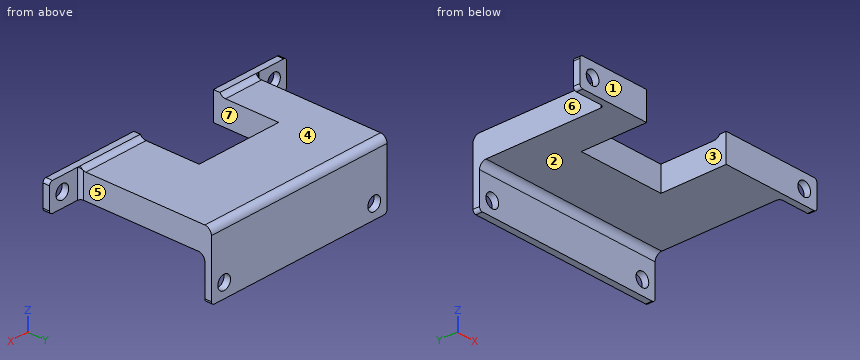
```python
from build123d import *

# Parameters (mm, degrees)
SKETCH1_W           = 79
SKETCH1_H           = 8.5
SKETCH1_R           = 2.125
BOSS_EXTRUDE1_DEPTH = 2
SKETCH3_W           = 58.5
SKETCH3_H           = 7.5
BOSS_EXTRUDE2_DEPTH = 40.14
SKETCH4_W           = 58.5
SKETCH4_H           = 2
BOSS_EXTRUDE3_DEPTH = 12.5
CUT_EXTRUDE1_REACH  = 93.966
SKETCH5_R           = 2.125
FILLET1_R           = 2
FILLET2_R           = 1
FILLET3_R           = 2
FILLET4_R           = 1
FILLET5_R           = 1
SKETCH6_W           = 26.5
SKETCH6_H           = 20
CUT_EXTRUDE2_DEPTH  = 10


with BuildPart() as part:
    # Sketch1 → Boss-Extrude1 (new body)
    with BuildSketch(Plane(origin=(0, 0, 0), x_dir=(1, 0, 0), z_dir=(0, 1, 0))):
        with Locations((-39.5, 4.25)):
            Rectangle(SKETCH1_W, SKETCH1_H)
        with Locations(Location((-74.75, 4.25, 0), (0, 0, 270))):
            Circle(SKETCH1_R, mode=Mode.SUBTRACT)
        with Locations(Location((-4.25, 4.25, 0), (0, 0, 270))):
            Circle(SKETCH1_R, mode=Mode.SUBTRACT)
    extrude(amount=BOSS_EXTRUDE1_DEPTH)

    # Sketch3 → Boss-Extrude2 (add)
    with BuildSketch(Plane(origin=(0, 2, 0), x_dir=(1, 0, 0), z_dir=(0, 1, 0))):
        with Locations((-39.5, 4.75)):
            Rectangle(SKETCH3_W, SKETCH3_H)
    extrude(amount=BOSS_EXTRUDE2_DEPTH)

    # Sketch4 → Boss-Extrude3 (add)
    with BuildSketch(Plane(origin=(0, 0, -8.5), x_dir=(-1, 0, 0), z_dir=(0, 0, -1))):
        with Locations((39.5, 41.14)):
            Rectangle(SKETCH4_W, SKETCH4_H)
    extrude(amount=BOSS_EXTRUDE3_DEPTH)

    # Sketch5 → Cut-Extrude1 (cut, up to next)
    with BuildSketch(Plane(origin=(0, 42.14, 0), x_dir=(1, 0, 0), z_dir=(0, 1, 0)), mode=Mode.PRIVATE) as cut_extrude1_sk1:
        with Locations(Location((-14.5, 16.75, 0), (0, 0, 270))):
            Circle(SKETCH5_R)
    cut_extrude1_tool1 = extrude(cut_extrude1_sk1.sketch, amount=-CUT_EXTRUDE1_REACH, mode=Mode.PRIVATE) & part.part
    # Sketch5 → Cut-Extrude1 (cut, up to next)
    with BuildSketch(Plane(origin=(0, 42.14, 0), x_dir=(1, 0, 0), z_dir=(0, 1, 0)), mode=Mode.PRIVATE) as cut_extrude1_sk2:
        with Locations(Location((-64.5, 16.75, 0), (0, 0, 270))):
            Circle(SKETCH5_R)
    cut_extrude1_tool2 = extrude(cut_extrude1_sk2.sketch, amount=-CUT_EXTRUDE1_REACH, mode=Mode.PRIVATE) & part.part
    add(cut_extrude1_tool1.solids().sort_by_distance((-14.5, 42.14, -16.75))[0], mode=Mode.SUBTRACT)
    add(cut_extrude1_tool2.solids().sort_by_distance((-64.5, 42.14, -16.75))[0], mode=Mode.SUBTRACT)

    # Fillet1
    # the kernel refuses this fillet: 2 mm, written as the material it adds along each edge
    with BuildSketch(Plane(origin=(-68.75, 40.14, -8.5), x_dir=(0, -1, 0), z_dir=(1, 0, 0))) as fillet1_piece_1:
        with BuildLine():
            CenterArc((FILLET1_R, FILLET1_R), FILLET1_R, 180, 90)
            Line((0, FILLET1_R), (-FILLET1_R * 0.02, FILLET1_R))
            Line((-FILLET1_R * 0.02, FILLET1_R), (-FILLET1_R * 0.02, -FILLET1_R * 0.02))
            Line((-FILLET1_R * 0.02, -FILLET1_R * 0.02), (FILLET1_R, -FILLET1_R * 0.02))
            Line((FILLET1_R, -FILLET1_R * 0.02), (FILLET1_R, 0))
        make_face()
    extrude(amount=58.5)
    with BuildSketch(Plane(origin=(-68.75, 2, -1), x_dir=(0, 0, 1), z_dir=(1, 0, 0))) as fillet1_piece_2:
        with BuildLine():
            CenterArc((2, -1.732050808), FILLET1_R, 120, 60)
            Line((0, -1.732050808), (-0.04, -1.732050808))
            Line((-0.04, -1.732050808), (-0.04, 0))
            Line((-0.04, 0), (0, 0.04))
            ThreePointArc((0, 0.04), (0.5, 0.04), (0.98, 0.034641016))
            Line((0.98, 0.034641016), (1, 0))
        make_face()
    extrude(amount=58.5)

    # Fillet2
    fillet2_edges = [part.edges().sort_by_distance(p)[0] for p in [
        (-79, 1, 0),
        (-79, 1, -8.5),
        (-68.75, 41.14, -21),
        (-10.25, 41.14, -21),
        (0, 1, -8.5),
        (0, 1, 0),
    ]]
    fillet(fillet2_edges, radius=FILLET2_R)

    # Fillet3
    fillet3_edges = [part.edges().sort_by_distance(p)[0] for p in [
        (-39.5, 42.14, -1),
    ]]
    fillet(fillet3_edges, radius=FILLET3_R)

    # Fillet4
    # the kernel refuses this fillet: 1 mm, written as the material it adds along each edge
    with BuildSketch(Plane(origin=(-10.25, 2, 0), x_dir=(0, 1, 0), z_dir=(0, 0, -1))) as fillet4_piece_1_section:
        with BuildLine():
            CenterArc((FILLET4_R, FILLET4_R), FILLET4_R, 180, 90)
            Line((0, FILLET4_R), (0, 0))
            Line((0, 0), (FILLET4_R, 0))
        make_face()
    fillet4_piece_1 = extrude(amount=8.5, mode=Mode.PRIVATE)
    fillet4_piece_1 = fillet4_piece_1 - Plane(origin=(-10.019982346, 3.732050808, 1), x_dir=(0, 0, 1), z_dir=(-1, 0, 0)) * Cylinder(2, 21, mode=Mode.PRIVATE)
    add(fillet4_piece_1)

    # Fillet5
    # the kernel refuses this fillet: 1 mm, written as the material it adds along each edge
    with BuildSketch(Plane(origin=(-68.75, 2, -8.5), x_dir=(-1, 0, 0), z_dir=(0, 0, 1))) as fillet5_piece_1_section:
        with BuildLine():
            CenterArc((FILLET5_R, -FILLET5_R), FILLET5_R, 90, 90)
            Line((0, -FILLET5_R), (0, 0))
            Line((0, 0), (FILLET5_R, 0))
        make_face()
    fillet5_piece_1 = extrude(amount=8.5, mode=Mode.PRIVATE)
    fillet5_piece_1 = fillet5_piece_1 - Plane(origin=(-68.980019627, 3.732050808, 1), x_dir=(0, 0, 1), z_dir=(-1, 0, 0)) * Cylinder(2, 21, mode=Mode.PRIVATE)
    add(fillet5_piece_1)

    # Sketch6 → Cut-Extrude2 (cut)
    with BuildSketch(Plane(origin=(0, 0, -8.5), x_dir=(-1, 0, 0), z_dir=(0, 0, -1))):
        with Locations((43.5, 10)):
            Rectangle(SKETCH6_W, SKETCH6_H)
    extrude(amount=-CUT_EXTRUDE2_DEPTH, mode=Mode.SUBTRACT)


solid = part.part
```
The model under review builds one solid part; all positions refer to its coordinate system, in mm. Face numbers are marked on the shaded views. A direction names the side the tool comes from. Give positions to 0.01 mm unless a question says otherwise; leave off trailing zeros. Write each loop counter-clockwise with the first axis right and the second up, starting at its lowest first coordinate (ties: lowest second). Pieces come first, ordered by that corner, then holes. Notation, with made-up numbers: M -38,36 L -31,36 A29 cw -31,63 Z; hole C -40,-4.5 d6. An arc over 180 degrees is marked long. Write each question's results on one line, items separated by ' | '. Start each with the question number.
1. We need section D-D (x = -14.5). Write out the cut boundary in (y, z) (3 decimals).
2. Mouldability with a two-part tool opening along X and no side actions: class the marked faces 4, 5, 6 and 7 as released by +X, released by -X, zero draft, split by the parting line, or undercut.
3. We need section C-C (x = -4.25). Write out the cut boundary in (y, z) (3 decimals).
4. Insertion check: pin 1 Ø3 at (x, z) = (-45.5, -14.5) entering from -Y; pin 2 Ø2 at (x, y) = (-28, 34.5) entering from +Z; pin 3 Ø4 at (x, z) = (-73, -2) entering from +Y; pin 4 Ø4 at (x, z) = (-74.75, -4.25) entering from +Y. Each pin has a flat end and moves straight along its axis. Give the tip position at first contact, or say it passes through.
5. We need section B-B (z = -4.25). Write out the cut boundary in (x, y) (3 decimals), and give its area (3 significant figures).
6. For probe 1 along X at (y, z) = (41.35, -16.75) (3 decimals); probe 2 along X at (y, z) = (0.5, -4.25) (3 decimals); probe 3 along X at (y, z) = (5, -4), list the stretches that pass through material, from the lowest coordinate up. Write a range as [from, to].
7. For the marked faces 1, 2 and 3, list the 3-axis set-ups (+Z, -Z, +X, -X, +Y, -Y) from which the entire face can be reached by the end or side of a thin tool; tool diameter is ignored.
8. We need section A-A (y = 6). Write out the cut boundary in (x, z), and give its area (3 significant figures).
Results found:
1) outline: M 0,-8.5 L 38.14,-8.5 A2 cw 40.14,-10.5 L 40.14,-14.625 L 42.14,-14.625 L 42.14,-3 A2 ccw 40.14,-1 L 3.732,-1 A2 cw 2,0 L 0,0 Z; M 40.14,-21 L 42.14,-21 L 42.14,-18.875 L 40.14,-18.875 Z
2) face 4: zero draft | face 5: released by +X | face 6: released by -X | face 7: undercut
3) outline: M 0,-8.5 L 2,-8.5 L 2,-6.375 L 0,-6.375 Z; M 0,-2.125 L 2,-2.125 L 2,0 L 0,0 Z
4) pin 1: stops at y = 40.14 | pin 2: stops at z = -1 | pin 3: stops at y = 2 | pin 4: passes through
5) outline: M -79,0 L -76.875,0 L -76.875,2 L -79,2 Z; M -72.625,0 L -56.75,0 L -56.75,20 L -30.25,20 L -30.25,0 L -6.375,0 L -6.375,2 L -9.25,2 A1 cw -10.25,3 L -10.25,42.14 L -68.75,42.14 L -68.75,3 A1 cw -69.75,2 L -72.625,2 Z; M -2.125,0 L 0,0 L 0,2 L -2.125,2 Z | area: 1,960 mm^2
6) probe 1: x = [-68.75, -66.625], [-62.375, -16.625], [-12.375, -10.25] | probe 2: x = [-79, -76.875], [-72.625, -56.75], [-30.25, -6.375], [-2.125, 0] | probe 3: x = [-68.75, -56.75], [-30.25, -10.25]
7) face 1: +Z, -Z, +X, -X, -Y | face 2: -Z, +X, -X, -Y | face 3: +Z, -Z, -Y
8) outline: M -68.75,-8.5 L -56.75,-8.5 L -56.75,-1 L -68.75,-1 Z; M -30.25,-8.5 L -10.25,-8.5 L -10.25,-1 L -30.25,-1 Z | area: 240 mm^2
